Verification items for the finished model (mm, model axes). Coordinates: 2 decimals unless noted, no trailing zeros. Order: outer loops, then holes, each group sorted by start corner. A loop starts at its lowest first (then second) coordinate and runs counter-clockwise, first axis right, second up. Notation, with made-up numbers: (-26, 69.25) -> (31, 69.25) arc R16 ccw to (31, 76.25) -> close; hole circle Ø3 at (65.5, -29.5). An arc over 180 degrees is marked (long way). Write each question's results on one line, items separated by ' | '. Start each with the question number.
(1) Thickness scan on probe 1 along X at (y, z) = (2.25, -109.5); probe 2 along X at (y, z) = (-2.75, -264.5); probe 3 along X at (y, z) = (5.75, -139) (3 decimals). Record the ranges inside material, lowest first. Write a range as [from, to].
(2) Cross-section at A-A on x = -4. Enter the section's corners in (y, z).
(3) Go/stop test with flat-tipped pins: pin 1 (8 mm diameter, centred on x = -19, z = -155, fed in from +Y); pin 2 (12 mm diameter, centred on x = -32, z = -211.5, fed in from +Y). Record where each tip stops, or that it passes through.
(4) Cross-section at B-B on z = -236. Give the number of separate pieces and of enclosed holes in the cut face, and give its area (3 significant figures).
```python
from build123d import *

# Parameters (mm, degrees)
SKETCH1_R      = 3.4
SKETCH1_R_2    = 3.400000006
EXTRUDE1_DEPTH = 300


with BuildPart() as part:
    # Sketch1 → Extrude1 (new body)
    with BuildSketch(Plane.XY):
        with BuildLine():
            Line((-36.828217803, 10), (-25.761678346, 10))
            ThreePointArc((-25.761678346, 10), (-24.566343162, 9.581217839), (-24.06, 8.420260776))
            Line((-24.06, 8.420260776), (-24.06, 7.505975062))
            ThreePointArc((-24.06, 7.505975062), (-24.567063435, 6.348506245), (-25.761678346, 5.936507937))
            Line((-25.761678346, 5.936507937), (-26.89856374, 5.936507937))
            Line((-26.89856374, 5.936507937), (-26.89856374, 6.405354551))
            Line((-26.89856374, 6.405354551), (-29.01515873, 6.405354551))
            ThreePointArc((-29.01515873, 6.405354551), (-29.913072103, 6.033426654), (-30.285, 5.135513281))
            Line((-30.285, 5.135513281), (-30.285, 2.878955078))
            ThreePointArc((-30.285, 2.878955078), (-30.217342047, 2.538803338), (-30.024667785, 2.250433031))
            Line((-30.024667785, 2.250433031), (-26.865511635, -0.908897163))
            ThreePointArc((-26.865511635, -0.908897163), (-25.324726136, -1.938463161), (-23.50722312, -2.3))
            Line((-23.50722312, -2.3), (-16.234679932, -2.3))
            ThreePointArc((-16.234679932, -2.3), (-14.417176915, -1.938463161), (-12.876391416, -0.908897163))
            Line((-12.876391416, -0.908897163), (-9.975332215, 1.992321863))
            ThreePointArc((-9.975332215, 1.992321863), (-9.782657953, 2.28069217), (-9.715, 2.620843911))
            Line((-9.715, 2.620843911), (-9.715, 5.135513281))
            ThreePointArc((-9.715, 5.135513281), (-10.086927897, 6.033426654), (-10.98484127, 6.405354551))
            Line((-10.98484127, 6.405354551), (-13.228511431, 6.405354551))
            Line((-13.228511431, 6.405354551), (-13.228511431, 5.936507937))
            Line((-13.228511431, 5.936507937), (-14.365396825, 5.936507937))
            ThreePointArc((-14.365396825, 5.936507937), (-15.478809408, 6.397698529), (-15.94, 7.511111111))
            Line((-15.94, 7.511111111), (-15.94, 8.425396825))
            ThreePointArc((-15.94, 8.425396825), (-15.478809408, 9.538809408), (-14.365396825, 10))
            Line((-14.365396825, 10), (-7.044126982, 10))
            Line((-7.044126982, 10), (14.552471996, 10))
            ThreePointArc((14.552471996, 10), (15.546813416, 9.477564883), (15.94, 8.425396825))
            Line((15.94, 8.425396825), (15.94, 7.511111111))
            ThreePointArc((15.94, 7.511111111), (15.478809408, 6.397698529), (14.365396825, 5.936507937))
            Line((14.365396825, 5.936507937), (13.228511431, 5.936507937))
            Line((13.228511431, 5.936507937), (13.228511431, 6.660633301))
            Line((13.228511431, 6.660633301), (10.98484127, 6.660633301))
            ThreePointArc((10.98484127, 6.660633301), (10.086927897, 6.288705404), (9.715, 5.390792031))
            Line((9.715, 5.390792031), (9.715, 3.134233829))
            ThreePointArc((9.715, 3.134233829), (9.782657953, 2.794082088), (9.975332215, 2.505711781))
            Line((9.975332215, 2.505711781), (13.134488365, -0.653618412))
            ThreePointArc((13.134488365, -0.653618412), (14.64473832, -1.821319739), (16.49277688, -2.3))
            Line((16.49277688, -2.3), (23.50722312, -2.3))
            ThreePointArc((23.50722312, -2.3), (25.324726136, -1.938463161), (26.865511635, -0.908897163))
            Line((26.865511635, -0.908897163), (30.024667785, 2.250433031))
            ThreePointArc((30.024667785, 2.250433031), (30.278278636, 2.655971567), (30.285, 3.134233829))
            Line((30.285, 3.134233829), (30.285, 5.390792031))
            ThreePointArc((30.285, 5.390792031), (29.913072103, 6.288705404), (29.01515873, 6.660633301))
            Line((29.01515873, 6.660633301), (26.771488569, 6.660633301))
            Line((26.771488569, 6.660633301), (26.771488569, 5.936507937))
            Line((26.771488569, 5.936507937), (25.634603175, 5.936507937))
            ThreePointArc((25.634603175, 5.936507937), (24.521190592, 6.397698529), (24.06, 7.511111111))
            Line((24.06, 7.511111111), (24.06, 8.425396825))
            ThreePointArc((24.06, 8.425396825), (24.453186584, 9.477564883), (25.447528004, 10))
            Line((25.447528004, 10), (33.075833554, 10))
            Line((33.075833554, 10), (36.885357363, 10))
            ThreePointArc((36.885357363, 10), (39.090491138, 9.050251023), (40, 6.828217785))
            Line((40, 6.828217785), (40, -6.828217785))
            ThreePointArc((40, -6.828217785), (39.069183486, -9.071177839), (36.825396825, -10))
            Line((36.825396825, -10), (-36.828217803, -10))
            ThreePointArc((-36.828217803, -10), (-39.071006503, -9.071006503), (-40, -6.828217803))
            Line((-40, -6.828217803), (-40, 6.828217803))
            ThreePointArc((-40, 6.828217803), (-39.071006503, 9.071006503), (-36.828217803, 10))
        make_face()
        with Locations((-34.004773868, -4)):
            Circle(SKETCH1_R, mode=Mode.SUBTRACT)
        with Locations(Location((34.004773868, -4, 0), (0, 0, 180))):
            Circle(SKETCH1_R_2, mode=Mode.SUBTRACT)
        with BuildLine():
            Line((-38.35, 2.595292927), (-38.35, 5.557055178))
            ThreePointArc((-38.35, 5.557055178), (-37.509428882, 7.554544736), (-35.493548116, 8.35))
            Line((-35.493548116, 8.35), (-32.569919859, 8.35))
            ThreePointArc((-32.569919859, 8.35), (-32.120963721, 8.164036279), (-31.935, 7.715080141))
            Line((-31.935, 7.715080141), (-31.935, 3.230213422))
            ThreePointArc((-31.935, 3.230213422), (-32.306927856, 2.332300148), (-33.20484113, 1.960372292))
            Line((-33.20484113, 1.960372292), (-37.715079365, 1.960372292))
            ThreePointArc((-37.715079365, 1.960372292), (-38.164036052, 2.14633624), (-38.35, 2.595292927))
        make_face(mode=Mode.SUBTRACT)
        with BuildLine():
            Line((13.450195503, -6.954394873), (-13.450195503, -6.954394873))
            ThreePointArc((-13.450195503, -6.954394873), (-14.036762187, -6.562412722), (-13.89908728, -5.870490687))
            Line((-13.89908728, -5.870490687), (-1.257767926, 6.769315833))
            ThreePointArc((-1.257767926, 6.769315833), (-1.051776589, 6.906937009), (-0.808800063, 6.955252915))
            Line((-0.808800063, 6.955252915), (0, 6.955204454))
            Line((0, 6.955204454), (0.808800063, 6.955252915))
            ThreePointArc((0.808800063, 6.955252915), (1.051776589, 6.906937009), (1.257767926, 6.769315833))
            Line((1.257767926, 6.769315833), (13.89908728, -5.870490687))
            ThreePointArc((13.89908728, -5.870490687), (14.036762187, -6.562412722), (13.450195503, -6.954394873))
        make_face(mode=Mode.SUBTRACT)
        with BuildLine():
            Line((35.554894965, 8.35), (32.563967874, 8.35))
            ThreePointArc((32.563967874, 8.35), (32.121226634, 8.164362109), (31.935, 7.721868186))
            Line((31.935, 7.721868186), (31.935, 3.245873842))
            ThreePointArc((31.935, 3.245873842), (32.306927897, 2.347960469), (33.20484127, 1.976032573))
            Line((33.20484127, 1.976032573), (37.680832198, 1.976032573))
            ThreePointArc((37.680832198, 1.976032573), (38.126707117, 2.122693703), (38.35, 2.535554718))
            Line((38.35, 2.535554718), (38.35, 5.496770698))
            ThreePointArc((38.35, 5.496770698), (37.552616332, 7.511327921), (35.554894965, 8.35))
        make_face(mode=Mode.SUBTRACT)
    extrude(amount=-EXTRUDE1_DEPTH)


solid = part.part
```
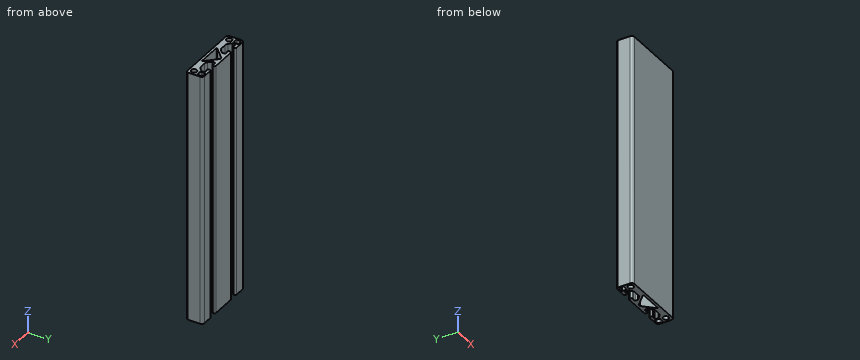
Results are:
1) probe 1: x = [-40, -38.25], [-32.4, -30.02], [-9.8, -5.78], [5.78, 10.23], [30.02, 32.42], [38.24, 40] | probe 2: x = [-40, -37.17], [-30.84, -10.78], [10.78, 30.84], [37.17, 40] | probe 3: x = [-40, -38.343], [-31.935, -30.126], [-9.874, -2.277], [2.277, 9.767], [30.233, 31.935], [38.344, 40]
2) outline: (-10, -300) -> (-6.95, -300) -> (-6.95, 0) -> (-10, 0) -> close; (4.03, -300) -> (10, -300) -> (10, 0) -> (4.03, 0) -> close
3) pin 1: stops at y = 9.87 | pin 2: stops at y = 10
4) separate pieces: 1 | enclosed holes: 5 | area: 851 mm2
